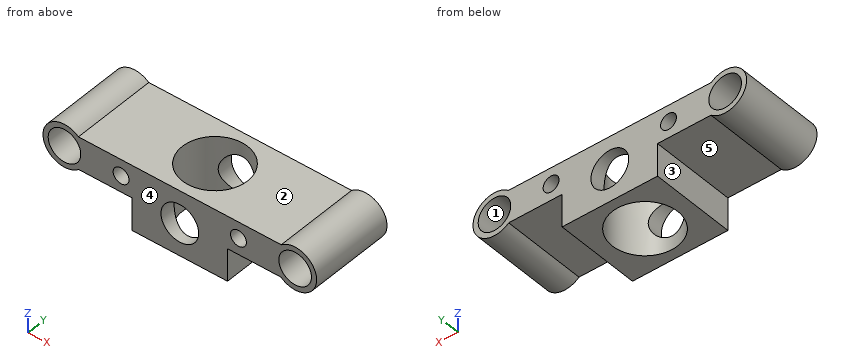
```python
from build123d import *

# Parameters (mm, degrees)
SKETCH002_R     = 2.5
PAD002_DEPTH    = 13
SKETCH_W        = 35
SKETCH_H        = 13
PAD_DEPTH       = 5
SKETCH003_R     = 3.3
PAD003_DEPTH    = 13
SKETCH005_W     = 14.63643
SKETCH005_H     = 13
PAD004_DEPTH    = 5
SKETCH004_R     = 5
POCKET_DEPTH    = 10.001
SKETCH006_R     = 2.893254
POCKET001_DEPTH = 13.001
SKETCH007_R     = 1.218023
POCKET002_DEPTH = 103.479644


with BuildPart() as pad002:
    # Sketch002 → Pad002 (new body)
    with BuildSketch(Plane.XZ.offset(6.5)):
        with Locations((17.683945, 2.483897)):
            Circle(SKETCH002_R)
    extrude(amount=-PAD002_DEPTH)


with BuildPart() as part_mirroring001:
    # Part__Mirroring001: instance of Pad002
    add(pad002.part.mirror(Plane(origin=(0, 0, 2.483897), x_dir=(0, -1, 0), z_dir=(1, 0, 0))))


with BuildPart() as scassi:
    # Fusion001 base: copy of Pad002
    add(pad002.part)

    # Fusion001: union Part__Mirroring001
    add(part_mirroring001.part)


with BuildPart() as cut:
    # Sketch → Pad (new body)
    with BuildSketch(Plane.XY):
        Rectangle(SKETCH_W, SKETCH_H)
    extrude(amount=PAD_DEPTH)

    # Sketch003 → Pad003 (new body)
    with BuildSketch(Plane.XZ.offset(6.5)):
        with Locations((17.683945, 2.483897)):
            Circle(SKETCH003_R)
        with Locations((-17.683945, 2.483897)):
            Circle(SKETCH003_R)
    extrude(amount=-PAD003_DEPTH)

    # Cut: cut scassi
    add(scassi.part, mode=Mode.SUBTRACT)


with BuildPart() as multitransform:
    # Sketch005 → Pad004 (new body)
    with BuildSketch(Plane(origin=(0, 0, 0), x_dir=(1, 0, 0), z_dir=(0, 0, -1))):
        Rectangle(SKETCH005_W, SKETCH005_H)
    extrude(amount=PAD004_DEPTH)

    # Fusion002: union Cut
    add(cut.part)

    # Sketch004 → Pocket (cut, through all)
    with BuildSketch(Plane.XY.offset(5)):
        Circle(SKETCH004_R)
    extrude(amount=-POCKET_DEPTH, mode=Mode.SUBTRACT)

    # Sketch006 → Pocket001 (cut, through all)
    with BuildSketch(Plane.XZ.offset(6.5)):
        Circle(SKETCH006_R)
    extrude(amount=-POCKET001_DEPTH, mode=Mode.SUBTRACT)

    # Sketch007 → Pocket002 (cut, through all)
    with BuildSketch(Plane.XZ.offset(6.5)):
        with Locations((9, 2.5)):
            Circle(SKETCH007_R)
    pocket002 = extrude(amount=-POCKET002_DEPTH, mode=Mode.SUBTRACT)

    # Mirrored: Pocket002 across Sketch007 V_Axis
    add(pocket002.mirror(Plane(origin=(0, -6.5, 0), x_dir=(0, -1, 0), z_dir=(1, 0, 0))), mode=Mode.SUBTRACT)


solid = multitransform.part
```
Work out the finished part from the listing and answer in its coordinate system (mm). Face numbers are marked on the shaded views. A direction names the side the tool comes from. Give positions to 0.01 mm unless a question says otherwise; leave off trailing zeros. Write each loop counter-clockwise with the first axis right and the second up, starting at its lowest first coordinate (ties: lowest second). Pieces come first, ordered by that corner, then holes.
(1) Which of the six approach directions +Z, -Z, +X, -X, +Y, -Y give full straight-line access (tool end or side, diameter ignored) to the marked faces 1, 2 and 3?
Final values:
face 1: +Y, -Y
face 2: +Z, +Y, -Y
face 3: -Z, +Y, -Y
(2) The part is cut by section D-D on z = -1.25. Write down the section's boundary in (x, y), plus the area to 3 significant figures.
Final values:
outline: (-7.32, -6.5) - (-2.61, -6.5) - (-2.61, -4.27) arc R5 cw to (-2.61, 4.27) - (-2.61, 6.5) - (-7.32, 6.5) - close; (2.61, -6.5) - (7.32, -6.5) - (7.32, 6.5) - (2.61, 6.5) - (2.61, 4.27) arc R5 cw to (2.61, -4.27) - close
area: 93.6 mm2
(3) Flat-ended cylindrical pins translate along their axes: pin 1 Ø3.5 at (x, z) = (0, 0) entering from -Y; pin 2 Ø4 at (y, z) = (-1.5, -2) entering from -X; pin 3 Ø4 at (y, z) = (-2, -3) entering from +X; pin 4 Ø5 at (x, y) = (-13, -3) entering from +Z. Find the tip coordinate at first contact, or state that the pin passes through.
Final values:
pin 1: passes through
pin 2: stops at x = -19.86
pin 3: stops at x = 7.32
pin 4: stops at z = 5
(4) The part is cut by section B-B on y = 2.5. Write down the section's boundary in (x, z).
Final values:
outline: (-15.55, 5) arc R3.3 ccw (long way) to (-15.51, 0) - (-7.32, 0) - (-7.32, -5) - (-4.33, -5) - (-4.33, 5) - close; (4.33, -5) - (7.32, -5) - (7.32, 0) - (15.51, 0) arc R3.3 ccw (long way) to (15.55, 5) - (4.33, 5) - close; hole circle Ø5 at (-17.68, 2.48); hole circle Ø2.44 at (-9, 2.5); hole circle Ø2.44 at (9, 2.5); hole circle Ø5 at (17.68, 2.48)
(5) The part is cut by section C-C on x = 0. Write down the section's boundary in (y, z).
Final values:
outline: (-6.5, -5) - (-5, -5) - (-5, -2.89) - (-6.5, -2.89) - close; (-6.5, 2.89) - (-5, 2.89) - (-5, 5) - (-6.5, 5) - close; (5, -5) - (6.5, -5) - (6.5, -2.89) - (5, -2.89) - close; (5, 2.89) - (6.5, 2.89) - (6.5, 5) - (5, 5) - close
(6) The mould has two halves that part along X. Classify the marked faces 4 and 5: pulls with the +X half, pulls with the -X half, needs draft (parallel to the pull), parting line crosses it, or undercut.
Final values:
face 4: needs draft
face 5: undercut
(7) The part is cut by section A-A on x = -9. Write down the section's boundary in (y, z), plus the area to 3 significant figures.
Final values:
outline: (-6.5, 0) - (6.5, 0) - (6.5, 1.28) - (-6.5, 1.28) - close; (-6.5, 3.72) - (6.5, 3.72) - (6.5, 5) - (-6.5, 5) - close
area: 33.3 mm2
(8) Straight lines are drawn through the part: line 1 (X direction, y = -0.25, z = -1); line 2 (X direction, y = -1.5, z = 4); line 3 (X direction, y = 2, z = 1). For each, find the intervals that lie inside material, in ascending order.
Final values:
line 1: x = -7.32 to -4.99, 4.99 to 7.32
line 2: x = -20.62 to -19.67, -15.7 to -4.77, 4.77 to 15.7, 19.67 to 20.62
line 3: x = -20.63 to -19.7, -15.67 to -4.58, 4.58 to 15.67, 19.7 to 20.63
